Autodesk Inventor part; units mm, degrees
ref_plane "YZ Plane" through (0, 0, 0) normal (1, 0, 0) x (0, 1, 0)
ref_plane "XZ Plane" through (0, 0, 0) normal (0, 1, 0) x (-1, 0, 0)
ref_plane "XY Plane" through (0, 0, 0) normal (0, 0, 1) x (1, 0, 0)
sketch "スケッチ1" plane through (0, 0, 0) normal (0, 1, 0) x (-1, 0, 0)
  line L0 (0, 0) -> (0, -30.5)
  line L1 (7.5, 2.25) -> (7.5, -32.75)
  line L2 (11.9991, -15.25) -> (-11.598, -15.25)
  line L3 (7.5, 2.25) -> (6.5, 2.25)
  line L4 (7.5, 2.25) -> (8.5, 2.25) construction
  line L5 (0, 0) -> (1, 0)
  arc A0 (1, 0) -> (6.5, 2.25) centre (3.2952, 2.2367) ccw
  line L6 (7.5, -32.75) -> (6.5, -32.75)
  line L7 (0, -30.5) -> (1, -30.5)
  arc A1 (6.5, -32.75) -> (1, -30.5) centre (3.2952, -32.7367) ccw
  line L8 (7.5, -2.15) -> (1, -2.15)
  line L9 (1, -2.15) -> (1, -28.35)
  line L10 (1, -28.35) -> (7.5, -28.35)
  dimension "d0" = 30.5
  dimension "d1" = 35
  dimension "d2" = 7.5
  dimension "d3" = 2.25
  dimension "d4" = 1
  dimension "d5" = 180
  dimension "d6" = 1
  dimension "d7" = 4.4
  dimension "d8" = 4.4
extrude "押し出し1" add sketch "スケッチ1" along normal blind 175 contours L5 A0 L3 L1 L8 L9 L2 L0 | L2 L9 L10 L1 L6 A1 L7 L0
sketch "スケッチ2" plane through (-1, 0, -28.35) normal (-1, 0, 0) x (0, 0, 1)
  line L0 (0, 0) -> (26.2, 0)
  line L1 (26.2, 0) -> (26.2, 175)
  line L2 (0, 175) -> (26.2, 175)
  line L3 (0, 0) -> (0, 175)
  line L4 (15.85, 3) -> (10.35, 3)
  line L5 (10.35, 3) -> (10.35, 11)
  line L6 (10.35, 11) -> (15.85, 11)
  line L7 (15.85, 11) -> (15.85, 3)
  arc A0 (13.1, 3) -> (15.85, 5.75) centre (13.1, 5.75) ccw
  arc A1 (10.35, 5.75) -> (13.1, 3) centre (13.1, 5.75) ccw
  arc A2 (13.1, 11) -> (10.35, 8.25) centre (13.1, 8.25) ccw
  arc A3 (15.85, 8.25) -> (13.1, 11) centre (13.1, 8.25) ccw
  line L8 (15.85, 15.5) -> (10.35, 15.5)
  arc A4 (13.1, 15.5) -> (15.85, 18.25) centre (13.1, 18.25) ccw
  arc A5 (10.35, 18.25) -> (13.1, 15.5) centre (13.1, 18.25) ccw
  arc A6 (15.85, 20.75) -> (13.1, 23.5) centre (13.1, 20.75) ccw
  arc A7 (13.1, 23.5) -> (10.35, 20.75) centre (13.1, 20.75) ccw
  line L9 (10.35, 15.5) -> (10.35, 23.5)
  line L10 (15.85, 23.5) -> (15.85, 15.5)
  line L11 (15.85, 28) -> (10.35, 28)
  arc A8 (13.1, 28) -> (15.85, 30.75) centre (13.1, 30.75) ccw
  arc A9 (10.35, 30.75) -> (13.1, 28) centre (13.1, 30.75) ccw
  arc A10 (15.85, 33.25) -> (13.1, 36) centre (13.1, 33.25) ccw
  arc A11 (13.1, 36) -> (10.35, 33.25) centre (13.1, 33.25) ccw
  line L12 (10.35, 28) -> (10.35, 36)
  line L13 (15.85, 36) -> (15.85, 28)
  line L14 (15.85, 40.5) -> (10.35, 40.5)
  arc A12 (13.1, 40.5) -> (15.85, 43.25) centre (13.1, 43.25) ccw
  arc A13 (10.35, 43.25) -> (13.1, 40.5) centre (13.1, 43.25) ccw
  arc A14 (15.85, 45.75) -> (13.1, 48.5) centre (13.1, 45.75) ccw
  arc A15 (13.1, 48.5) -> (10.35, 45.75) centre (13.1, 45.75) ccw
  line L15 (10.35, 40.5) -> (10.35, 48.5)
  line L16 (15.85, 48.5) -> (15.85, 40.5)
  line L17 (15.85, 53) -> (10.35, 53)
  arc A16 (13.1, 53) -> (15.85, 55.75) centre (13.1, 55.75) ccw
  arc A17 (10.35, 55.75) -> (13.1, 53) centre (13.1, 55.75) ccw
  arc A18 (15.85, 58.25) -> (13.1, 61) centre (13.1, 58.25) ccw
  arc A19 (13.1, 61) -> (10.35, 58.25) centre (13.1, 58.25) ccw
  line L18 (10.35, 53) -> (10.35, 61)
  line L19 (15.85, 61) -> (15.85, 53)
  line L20 (15.85, 65.5) -> (10.35, 65.5)
  arc A20 (13.1, 65.5) -> (15.85, 68.25) centre (13.1, 68.25) ccw
  arc A21 (10.35, 68.25) -> (13.1, 65.5) centre (13.1, 68.25) ccw
  arc A22 (15.85, 70.75) -> (13.1, 73.5) centre (13.1, 70.75) ccw
  arc A23 (13.1, 73.5) -> (10.35, 70.75) centre (13.1, 70.75) ccw
  line L21 (10.35, 65.5) -> (10.35, 73.5)
  line L22 (15.85, 73.5) -> (15.85, 65.5)
  line L23 (15.85, 78) -> (10.35, 78)
  arc A24 (13.1, 78) -> (15.85, 80.75) centre (13.1, 80.75) ccw
  arc A25 (10.35, 80.75) -> (13.1, 78) centre (13.1, 80.75) ccw
  arc A26 (15.85, 83.25) -> (13.1, 86) centre (13.1, 83.25) ccw
  arc A27 (13.1, 86) -> (10.35, 83.25) centre (13.1, 83.25) ccw
  line L24 (10.35, 78) -> (10.35, 86)
  line L25 (15.85, 86) -> (15.85, 78)
  line L26 (15.85, 90.5) -> (10.35, 90.5)
  arc A28 (13.1, 90.5) -> (15.85, 93.25) centre (13.1, 93.25) ccw
  arc A29 (10.35, 93.25) -> (13.1, 90.5) centre (13.1, 93.25) ccw
  arc A30 (15.85, 95.75) -> (13.1, 98.5) centre (13.1, 95.75) ccw
  arc A31 (13.1, 98.5) -> (10.35, 95.75) centre (13.1, 95.75) ccw
  line L27 (10.35, 90.5) -> (10.35, 98.5)
  line L28 (15.85, 98.5) -> (15.85, 90.5)
  line L29 (15.85, 103) -> (10.35, 103)
  arc A32 (13.1, 103) -> (15.85, 105.75) centre (13.1, 105.75) ccw
  arc A33 (10.35, 105.75) -> (13.1, 103) centre (13.1, 105.75) ccw
  arc A34 (15.85, 108.25) -> (13.1, 111) centre (13.1, 108.25) ccw
  arc A35 (13.1, 111) -> (10.35, 108.25) centre (13.1, 108.25) ccw
  line L30 (10.35, 103) -> (10.35, 111)
  line L31 (15.85, 111) -> (15.85, 103)
  line L32 (15.85, 115.5) -> (10.35, 115.5)
  arc A36 (13.1, 115.5) -> (15.85, 118.25) centre (13.1, 118.25) ccw
  arc A37 (10.35, 118.25) -> (13.1, 115.5) centre (13.1, 118.25) ccw
  arc A38 (15.85, 120.75) -> (13.1, 123.5) centre (13.1, 120.75) ccw
  arc A39 (13.1, 123.5) -> (10.35, 120.75) centre (13.1, 120.75) ccw
  line L33 (10.35, 115.5) -> (10.35, 123.5)
  line L34 (15.85, 123.5) -> (15.85, 115.5)
  line L35 (15.85, 128) -> (10.35, 128)
  arc A40 (13.1, 128) -> (15.85, 130.75) centre (13.1, 130.75) ccw
  arc A41 (10.35, 130.75) -> (13.1, 128) centre (13.1, 130.75) ccw
  arc A42 (15.85, 133.25) -> (13.1, 136) centre (13.1, 133.25) ccw
  arc A43 (13.1, 136) -> (10.35, 133.25) centre (13.1, 133.25) ccw
  line L36 (10.35, 128) -> (10.35, 136)
  line L37 (15.85, 136) -> (15.85, 128)
  line L38 (15.85, 140.5) -> (10.35, 140.5)
  arc A44 (13.1, 140.5) -> (15.85, 143.25) centre (13.1, 143.25) ccw
  arc A45 (10.35, 143.25) -> (13.1, 140.5) centre (13.1, 143.25) ccw
  arc A46 (15.85, 145.75) -> (13.1, 148.5) centre (13.1, 145.75) ccw
  arc A47 (13.1, 148.5) -> (10.35, 145.75) centre (13.1, 145.75) ccw
  line L39 (10.35, 140.5) -> (10.35, 148.5)
  line L40 (15.85, 148.5) -> (15.85, 140.5)
  line L41 (15.85, 153) -> (10.35, 153)
  arc A48 (13.1, 153) -> (15.85, 155.75) centre (13.1, 155.75) ccw
  arc A49 (10.35, 155.75) -> (13.1, 153) centre (13.1, 155.75) ccw
  arc A50 (15.85, 158.25) -> (13.1, 161) centre (13.1, 158.25) ccw
  arc A51 (13.1, 161) -> (10.35, 158.25) centre (13.1, 158.25) ccw
  line L42 (10.35, 153) -> (10.35, 161)
  line L43 (15.85, 161) -> (15.85, 153)
  line L44 (15.85, 165.5) -> (10.35, 165.5)
  arc A52 (13.1, 165.5) -> (15.85, 168.25) centre (13.1, 168.25) ccw
  arc A53 (10.35, 168.25) -> (13.1, 165.5) centre (13.1, 168.25) ccw
  arc A54 (15.85, 170.75) -> (13.1, 173.5) centre (13.1, 170.75) ccw
  arc A55 (13.1, 173.5) -> (10.35, 170.75) centre (13.1, 170.75) ccw
  line L45 (10.35, 165.5) -> (10.35, 173.5)
  line L46 (15.85, 173.5) -> (15.85, 165.5)
  line L47 (15.85, 178) -> (10.35, 178)
  arc A56 (13.1, 178) -> (15.85, 180.75) centre (13.1, 180.75) ccw
  arc A57 (10.35, 180.75) -> (13.1, 178) centre (13.1, 180.75) ccw
  arc A58 (15.85, 183.25) -> (13.1, 186) centre (13.1, 183.25) ccw
  arc A59 (13.1, 186) -> (10.35, 183.25) centre (13.1, 183.25) ccw
  line L48 (10.35, 178) -> (10.35, 186)
  line L49 (15.85, 186) -> (15.85, 178)
  line L50 (15.85, 190.5) -> (10.35, 190.5)
  arc A60 (13.1, 190.5) -> (15.85, 193.25) centre (13.1, 193.25) ccw
  arc A61 (10.35, 193.25) -> (13.1, 190.5) centre (13.1, 193.25) ccw
  arc A62 (15.85, 195.75) -> (13.1, 198.5) centre (13.1, 195.75) ccw
  arc A63 (13.1, 198.5) -> (10.35, 195.75) centre (13.1, 195.75) ccw
  line L51 (10.35, 190.5) -> (10.35, 198.5)
  line L52 (15.85, 198.5) -> (15.85, 190.5)
  line L53 (15.85, 203) -> (10.35, 203)
  arc A64 (13.1, 203) -> (15.85, 205.75) centre (13.1, 205.75) ccw
  arc A65 (10.35, 205.75) -> (13.1, 203) centre (13.1, 205.75) ccw
  arc A66 (15.85, 208.25) -> (13.1, 211) centre (13.1, 208.25) ccw
  arc A67 (13.1, 211) -> (10.35, 208.25) centre (13.1, 208.25) ccw
  line L54 (10.35, 203) -> (10.35, 211)
  line L55 (15.85, 211) -> (15.85, 203)
  line L56 (15.85, 215.5) -> (10.35, 215.5)
  arc A68 (13.1, 215.5) -> (15.85, 218.25) centre (13.1, 218.25) ccw
  arc A69 (10.35, 218.25) -> (13.1, 215.5) centre (13.1, 218.25) ccw
  arc A70 (15.85, 220.75) -> (13.1, 223.5) centre (13.1, 220.75) ccw
  arc A71 (13.1, 223.5) -> (10.35, 220.75) centre (13.1, 220.75) ccw
  line L57 (10.35, 215.5) -> (10.35, 223.5)
  line L58 (15.85, 223.5) -> (15.85, 215.5)
  line L59 (15.85, 228) -> (10.35, 228)
  arc A72 (13.1, 228) -> (15.85, 230.75) centre (13.1, 230.75) ccw
  arc A73 (10.35, 230.75) -> (13.1, 228) centre (13.1, 230.75) ccw
  arc A74 (15.85, 233.25) -> (13.1, 236) centre (13.1, 233.25) ccw
  arc A75 (13.1, 236) -> (10.35, 233.25) centre (13.1, 233.25) ccw
  line L60 (10.35, 228) -> (10.35, 236)
  line L61 (15.85, 236) -> (15.85, 228)
  line L62 (15.85, 240.5) -> (10.35, 240.5)
  arc A76 (13.1, 240.5) -> (15.85, 243.25) centre (13.1, 243.25) ccw
  arc A77 (10.35, 243.25) -> (13.1, 240.5) centre (13.1, 243.25) ccw
  arc A78 (15.85, 245.75) -> (13.1, 248.5) centre (13.1, 245.75) ccw
  arc A79 (13.1, 248.5) -> (10.35, 245.75) centre (13.1, 245.75) ccw
  line L63 (10.35, 240.5) -> (10.35, 248.5)
  line L64 (15.85, 248.5) -> (15.85, 240.5)
  line L65 (15.85, 253) -> (10.35, 253)
  arc A80 (13.1, 253) -> (15.85, 255.75) centre (13.1, 255.75) ccw
  arc A81 (10.35, 255.75) -> (13.1, 253) centre (13.1, 255.75) ccw
  arc A82 (15.85, 258.25) -> (13.1, 261) centre (13.1, 258.25) ccw
  arc A83 (13.1, 261) -> (10.35, 258.25) centre (13.1, 258.25) ccw
  line L66 (10.35, 253) -> (10.35, 261)
  line L67 (15.85, 261) -> (15.85, 253)
  line L68 (15.85, 265.5) -> (10.35, 265.5)
  arc A84 (13.1, 265.5) -> (15.85, 268.25) centre (13.1, 268.25) ccw
  arc A85 (10.35, 268.25) -> (13.1, 265.5) centre (13.1, 268.25) ccw
  arc A86 (15.85, 270.75) -> (13.1, 273.5) centre (13.1, 270.75) ccw
  arc A87 (13.1, 273.5) -> (10.35, 270.75) centre (13.1, 270.75) ccw
  line L69 (10.35, 265.5) -> (10.35, 273.5)
  line L70 (15.85, 273.5) -> (15.85, 265.5)
  line L71 (15.85, 278) -> (10.35, 278)
  arc A88 (13.1, 278) -> (15.85, 280.75) centre (13.1, 280.75) ccw
  arc A89 (10.35, 280.75) -> (13.1, 278) centre (13.1, 280.75) ccw
  arc A90 (15.85, 283.25) -> (13.1, 286) centre (13.1, 283.25) ccw
  arc A91 (13.1, 286) -> (10.35, 283.25) centre (13.1, 283.25) ccw
  line L72 (10.35, 278) -> (10.35, 286)
  line L73 (15.85, 286) -> (15.85, 278)
  line L74 (15.85, 290.5) -> (10.35, 290.5)
  arc A92 (13.1, 290.5) -> (15.85, 293.25) centre (13.1, 293.25) ccw
  arc A93 (10.35, 293.25) -> (13.1, 290.5) centre (13.1, 293.25) ccw
  arc A94 (15.85, 295.75) -> (13.1, 298.5) centre (13.1, 295.75) ccw
  arc A95 (13.1, 298.5) -> (10.35, 295.75) centre (13.1, 295.75) ccw
  line L75 (10.35, 290.5) -> (10.35, 298.5)
  line L76 (15.85, 298.5) -> (15.85, 290.5)
  line L77 (15.85, 303) -> (10.35, 303)
  arc A96 (13.1, 303) -> (15.85, 305.75) centre (13.1, 305.75) ccw
  arc A97 (10.35, 305.75) -> (13.1, 303) centre (13.1, 305.75) ccw
  arc A98 (15.85, 308.25) -> (13.1, 311) centre (13.1, 308.25) ccw
  arc A99 (13.1, 311) -> (10.35, 308.25) centre (13.1, 308.25) ccw
  line L78 (10.35, 303) -> (10.35, 311)
  line L79 (15.85, 311) -> (15.85, 303)
  point P0 (28.35, 0)
  dimension "d11" = 5.5
  dimension "d12" = 8
  dimension "d13" = 10.35
  dimension "d14" = 3
  dimension "d16" = 2.75
  dimension "d18" = 2.75
  dimension "d21" = 12.5
extrude "押し出し2" cut sketch "スケッチ2" against normal blind 3 contours A1 L5 A2 A3 L7 A0 | A5 L9 A7 A6 L10 A4 | A9 L12 A11 A10 L13 A8 | A13 L15 A15 A14 L16 A12 | A17 L18 A19 A18 L19 A16 | A21 L21 A23 A22 L22 A20 | A25 L24 A27 A26 L25 A24 | A29 L27 A31 A30 L28 A28 | A33 L30 A35 A34 L31 A32 | A37 L33 A39 A38 L34 A36 | A41 L36 A43 A42 L37 A40 | A45 L39 A47 A46 L40 A44 | A49 L42 A51 A50 L43 A48 | A53 L45 A55 A54 L46 A52 | A57 L48 A59 A58 L49 A56 | A61 L51 A63 A62 L52 A60 | A65 L54 A67 A66 L55 A64 | A69 L57 A71 A70 L58 A68 | A73 L60 A75 A74 L61 A72 | A77 L63 A79 A78 L64 A76 | A81 L66 A83 A82 L67 A80 | A85 L69 A87 A86 L70 A84 | A89 L72 A91 A90 L73 A88 | A93 L75 A95 A94 L76 A92
fillet "フィレット1" radius 1 2 edges at (-1, 87.5, -28.35) (-1, 87.5, -2.15)
properties part number "CB_dinrail_mk" material "アルミニウム 6061-AHC"
Geometry check sheet. Reference: the model listing, model coordinates, mm. A direction names the side the tool comes from. Give positions to 0.01 mm unless a question says otherwise; leave off trailing zeros. Loops run counter-clockwise (first coordinate to the right, second up) from the corner with the lowest first, then second, coordinate; pieces in that order, holes last. Notation, with made-up numbers: (55.5, 74) -> (106.5, 74) arc R34 ccw to (106.5, 111) -> close; hole circle Ø10 at (23.5, 71.5). An arc over 180 degrees is marked (long way). Answer in a Markdown table with one row per item. Add a question column.
1) Cross-section at B-B on z = -15.25. State how many separate pieces and enclosed holes the cut face has, and give its area (3 significant figures).
2) Material ranges on probe 1 along Z at (x, y) = (-3, 138.5); probe 2 along X at (y, z) = (139, -15); probe 3 along Z at (x, y) = (-1.25, 41), recorded low to high. Write a range as from..to.
3) Cross-section at C-C on z = -22. Record the boundary of the cut face in (x, y).
4) Set-up check for faces 4 (the face through (-7.5, 86, 0)), 5 (the face through (-0.5, 140.5, -15.3)), 6 (the face through (-5, 86, -2.15)): record each of +Z, -Z, +X, -X, +Y, -Y from which the full face is reachable in a straight line by a thin tool's end or side.
5) Draft check along Y on faces 1 (the face through (-1, 86.3, -15.1)), 2 (the face through (-0.5, 111, -15.2)), 3 (the face through (-0.7, 175, -15.2)). Enter one of: pulls with the +Y half, pulls with the -Y half, needs draft (parallel to the pull), parting line crosses it, or undercut.
6) Cross-section at A-A on x = -5.25. Record the boundary of the cut face in (y, z), and give its area (3 significant figures).
7) Gauge pin test, flat ends, axial feed: P1, Ø1.1, axis at x = -0.5, y = 45, coming from the +Z side; P2, Ø1.1, axis at x = -0.5, y = 169.5, coming from the -Z side; P3, Ø10, axis at y = 137, z = -11, coming from the -X side; P4, Ø4, axis at x = -6, y = 96, coming from the -Z side. Record the tip position at first contact, or that the pin passes through.
Outcome:
| question | item | result |
|---|---|---|
| 1 | separate pieces | 15 |
| 1 | enclosed holes | 0 |
| 1 | area | 63.0 mm^2 |
| 2 | probe 1 | z = -29.55..-28.35, -2.15..-0.95 |
| 2 | probe 2 | x = -1..0 |
| 2 | probe 3 | z = -30.27..-28.01, -2.49..-0.23 |
| 3 | outline | (-1, 0) -> (0, 0) -> (0, 175) -> (-1, 175) -> close |
| 4 | face 4 | +Z, -Z, -X, +Y, -Y |
| 4 | face 5 | +X, -X |
| 4 | face 6 | -X, +Y, -Y |
| 5 | face 1 | needs draft |
| 5 | face 2 | undercut |
| 5 | face 3 | pulls with the +Y half |
| 6 | outline | (0, -30.2) -> (175, -30.2) -> (175, -28.35) -> (0, -28.35) -> close; (0, -2.15) -> (175, -2.15) -> (175, -0.3) -> (0, -0.3) -> close |
| 6 | area | 646 mm^2 |
| 7 | P1 | stops at z = 0 |
| 7 | P2 | stops at z = -30.5 |
| 7 | P3 | stops at x = -1 |
| 7 | P4 | stops at z = -32.75 |
